Read the model definition and answer for the solid it produces. Units are mm, in the model's axes. Face numbers are marked on the shaded views. A direction names the side the tool comes from. Give positions to 0.01 mm unless a question says otherwise; leave off trailing zeros. Write each loop counter-clockwise with the first axis right and the second up, starting at its lowest first coordinate (ties: lowest second). Pieces come first, ordered by that corner, then holes. Notation, with made-up numbers: M 21,9 L 67,9 A30 cw 67,33 Z; hole C 30,16 d4. An arc over 180 degrees is marked long. Write each question's results on one line, items separated by ' | '. Start each with the question number.
```python
from build123d import *

# Parameters (mm, degrees)
PAD_DEPTH       = 74
POCKET_DEPTH    = 5
SKETCH001_R     = 9.5
POCKET001_DEPTH = 67
FILLET_R        = 20
FILLET001_R     = 2
FILLET002_R     = 20
FILLET003_R     = 2
SKETCH014_W     = 7.96524
SKETCH014_H     = 15.164599
POCKET005_DEPTH = 5


with BuildPart() as part:
    # Sketch002 → Pad (new body)
    with BuildSketch(Plane.XY):
        with BuildLine():
            Line((0, 21), (46.6148, 21))
            ThreePointArc((46.64809, 0), (62.821811, 10.525666), (46.6148, 21))
            Line((46.64809, 0), (0, 0))
            Line((0, 0), (0, 21))
        make_face()
    extrude(amount=PAD_DEPTH)

    # Sketch → Pocket (cut)
    with BuildSketch(Plane.XY.offset(74)):
        with BuildLine():
            Line((1.502029, 1.496604), (48.477029, 1.496604))
            ThreePointArc((48.477029, 1.496604), (61.01841, 10.496604), (48.477029, 19.496604))
            Line((1.502029, 19.496604), (48.477029, 19.496604))
            Line((1.502029, 19.496604), (1.502029, 1.496604))
        make_face()
    extrude(amount=-POCKET_DEPTH, mode=Mode.SUBTRACT)

    # Sketch001 → Pocket001 (cut)
    with BuildSketch(Plane.XY.offset(69)):
        with Locations((51.354257, 10.5)):
            Circle(SKETCH001_R)
        Polygon((1.487366, 19.5069), (40.487343, 19.54915), (40.471612, 12.505767), (39.471612, 12.504684), (39.504804, 1.504734), (2.504921, 1.504734), (2.471729, 12.504684), (1.471732, 12.506917), align=None)
    extrude(amount=-POCKET001_DEPTH, mode=Mode.SUBTRACT)

    # Fillet
    fillet_edges = [part.edges().sort_by_distance(p)[0] for p in [
        (46.6148, 21, 37),
    ]]
    fillet(fillet_edges, radius=FILLET_R)

    # Fillet001
    fillet001_edges = [part.edges().sort_by_distance(p)[0] for p in [
        (0, 21, 37),
    ]]
    fillet(fillet001_edges, radius=FILLET001_R)

    # Fillet002
    fillet002_edges = [part.edges().sort_by_distance(p)[0] for p in [
        (46.64809, 0, 37),
    ]]
    fillet(fillet002_edges, radius=FILLET002_R)

    # Fillet003
    fillet003_edges = [part.edges().sort_by_distance(p)[0] for p in [
        (0, 0, 37),
    ]]
    fillet(fillet003_edges, radius=FILLET003_R)

    # Sketch014 → Pocket005 (cut)
    with BuildSketch(Plane.XY.offset(69)):
        with Locations((42.834709, 10.705082)):
            Rectangle(SKETCH014_W, SKETCH014_H)
    extrude(amount=-POCKET005_DEPTH, mode=Mode.SUBTRACT)


solid = part.part
```
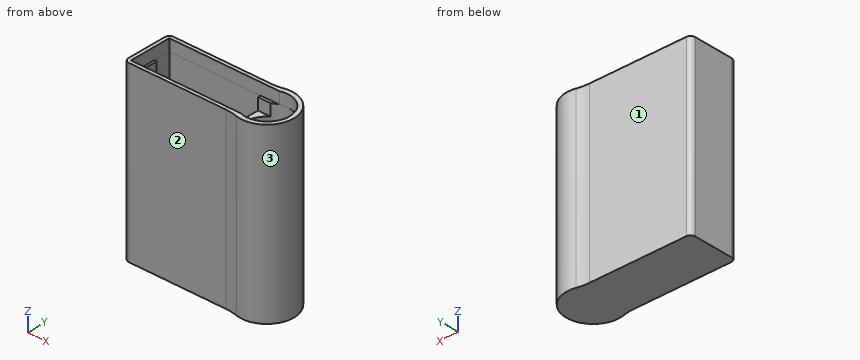
Item 1: Straight lines are drawn through the part: line 1 (X direction, y = 10.5, z = 30); line 2 (Y direction, x = 35, z = 68); line 3 (X direction, y = 7.75, z = 19.5). For each, find the intervals that lie inside material, in ascending order.
Item 2: Section C-C, the plane y = 9 is taken. Determine the outline of the cut face in (x, z).
Item 3: Section A-A, the plane z = 47.5 is taken. Determine the outline of the cut face in (x, y).
Item 4: Given P1, Ø8, axis at x = 23.5, z = 16, coming from the +Y side; P2, Ø2, axis at y = 17.5, z = 49.5, coming from the +X side; P3, Ø12.5, axis at x = 31, z = 25.5, coming from the -Y side, each flat-ended and moving along its own axis, determine where each tip first touches the part or whether it passes through.
Item 5: For the marked faces 1, 2 and 3, determine the directions among +Z, -Z, +X, -X, +Y, -Y from which every point of the face is accessible in a straight line to the end or side of a thin tool.
Worked out:
1) line 1: x = 0 to 2.48, 39.48 to 41.85, 60.85 to 62.82 | line 2: y = 0 to 1.5, 19.54 to 21 | line 3: x = 0 to 2.49, 39.49 to 42.26, 60.45 to 62.49
2) outline: M 0,0 L 62.72,0 L 62.72,74 L 60.9,74 L 60.9,69 L 60.74,69 L 60.74,2 L 41.97,2 L 41.97,64 L 39.48,64 L 39.48,2 L 2.48,2 L 2.48,69 L 1.5,69 L 1.5,74 L 0,74 Z
3) outline: M 0,2 A2 ccw 2,0 L 43.48,0 A20 cw 48.46,-0.63 A11.5 ccw long 48.44,21.64 A20 cw 43.42,21 L 2,21 A2 ccw 0,19 Z; hole M 1.47,12.51 L 2.47,12.5 L 2.5,1.5 L 39.5,1.5 L 39.47,12.5 L 40.47,12.51 L 40.49,19.55 L 1.49,19.51 Z; hole C 51.35,10.5 d19
4) P1: stops at y = 21 | P2: stops at x = 61.14 | P3: stops at y = 0
5) face 1: +Z, -Z, -X, +Y | face 2: +Z, -Z, -X, -Y | face 3: +Z, -Z
